Check sheet for the modelled part. Datum: model origin and axes. Units: mm. A direction names the side the tool comes from. Give positions to 0.01 mm unless a question says otherwise; leave off trailing zeros. Loops run counter-clockwise (first coordinate to the right, second up) from the corner with the lowest first, then second, coordinate; pieces in that order, holes last. Notation, with made-up numbers: M 24.5,29.25 L 56.5,29.25 A9 cw 56.5,38.25 Z; hole C -16,9.25 d5. An arc over 180 degrees is marked long. One line per question, with ' | ' between items. Start each with the question number.
from build123d import *

# Parameters (mm, degrees)
SKETCH1_W              = 127
SKETCH1_H              = 111.76
BASE_FLANGE1_DEPTH     = 1.5875
SKETCHED_START         = -63.5
SKETCHED_BEND1_DEPTH   = 127
SKETCHED_BEND1_2_DEPTH = 127
CUT_EXTRUDE2_START     = -2.3241
CUT_EXTRUDE2_OUTLINE_W = 17.78
CUT_EXTRUDE2_OUTLINE_H = 84
CUT_EXTRUDE2_DEPTH     = 2.3241
CUT_EXTRUDE1_REACH     = 106.317
SKETCH6_R              = 3.96875
CUT_EXTRUDE3_DEPTH     = 78.328235904
SKETCH34_W             = 31.75
SKETCH34_H             = 73.025
CUT_EXTRUDE5_DEPTH     = 2.54
CUT_EXTRUDE6_REACH     = 106.317
SKETCH49_W             = 17.78
SKETCH49_H             = 2.54


# Read off the part's stored shape, not the designer's step: Sketched Bend1, Cut-Extrude2
# Sheet-metal steps are written as plain solids
with BuildPart() as part:
    # Sketch1 → Base-Flange1 (new body)
    with BuildSketch(Plane.XY):
        Rectangle(SKETCH1_W, SKETCH1_H)
    extrude(amount=-BASE_FLANGE1_DEPTH)

    # Sketched Bend1 outline → Sketched Bend1 (cut)
    with BuildSketch(Plane.YZ.offset(SKETCHED_START)):
        with BuildLine():
            ThreePointArc((38.1, 0), (39.458217352, -0.438182071), (40.304282479, -1.5875))
            Line((40.304282479, -1.5875), (55.88, -1.5875))
            Line((55.88, -1.5875), (55.88, 0))
            Line((55.88, 0), (38.1, 0))
        make_face()
        with BuildLine():
            Line((-55.88, -1.5875), (-40.304282479, -1.5875))
            ThreePointArc((-40.304282479, -1.5875), (-39.458217352, -0.438182071), (-38.1, 0))
            Line((-38.1, 0), (-55.88, 0))
            Line((-55.88, 0), (-55.88, -1.5875))
        make_face()
    extrude(amount=SKETCHED_BEND1_DEPTH, mode=Mode.SUBTRACT)

    # Sketched Bend1 2 outline → Sketched Bend1 2 (add)
    with BuildSketch(Plane.YZ.offset(SKETCHED_START)):
        with BuildLine():
            ThreePointArc((38.1, -1.5875), (38.620854855, -1.803245145), (38.8366, -2.3241))
            Line((38.8366, -2.3241), (38.8366, -17.700231841))
            Line((38.8366, -17.700231841), (40.4241, -17.700231841))
            Line((40.4241, -17.700231841), (40.4241, -2.3241))
            ThreePointArc((40.4241, -2.3241), (40.393950056, -1.950959343), (40.304282479, -1.5875))
            Line((40.304282479, -1.5875), (38.1, -1.5875))
        make_face()
        with BuildLine():
            ThreePointArc((-38.8366, -2.3241), (-38.620854855, -1.803245145), (-38.1, -1.5875))
            Line((-38.1, -1.5875), (-40.304282479, -1.5875))
            ThreePointArc((-40.304282479, -1.5875), (-40.393950056, -1.950959343), (-40.4241, -2.3241))
            Line((-40.4241, -2.3241), (-40.4241, -17.700231841))
            Line((-40.4241, -17.700231841), (-38.8366, -17.700231841))
            Line((-38.8366, -17.700231841), (-38.8366, -2.3241))
        make_face()
    extrude(amount=SKETCHED_BEND1_2_DEPTH)

    # Cut-Extrude2 outline → Cut-Extrude2 (cut)
    with BuildSketch(Plane.XY.offset(CUT_EXTRUDE2_START)):
        with Locations((54.61, 0)):
            Rectangle(CUT_EXTRUDE2_OUTLINE_W, CUT_EXTRUDE2_OUTLINE_H)
    extrude(amount=CUT_EXTRUDE2_DEPTH, mode=Mode.SUBTRACT)

    # Cut-Extrude1: up to this face of the body (flat: up to its plane)
    cut_extrude1_end = Plane(part.part.faces().sort_by_distance((0, -40.4241, -10.012165921))[0])
    # Sketch6 → Cut-Extrude1 (cut, up to the picked face)
    with BuildSketch(Plane(origin=(0, 40.4241, 0), x_dir=(1, 0, 0), z_dir=(0, 1, 0)), mode=Mode.PRIVATE) as cut_extrude1_sk1:
        with Locations(Location((56.515, 10.4775, 0), (0, 0, 270))):
            Circle(SKETCH6_R)
    cut_extrude1_tool1 = split(extrude(cut_extrude1_sk1.sketch, amount=-CUT_EXTRUDE1_REACH, mode=Mode.PRIVATE), bisect_by=cut_extrude1_end, keep=Keep.BOTH, mode=Mode.PRIVATE)
    add(cut_extrude1_tool1.solids().sort_by(Axis((56.515, 40.4241, -10.4775), (0, -1, 0)))[0], mode=Mode.SUBTRACT)

    # Sketch13 → Cut-Extrude3 (cut, through all)
    with BuildSketch(Plane.XY):
        with BuildLine():
            ThreePointArc((45.72, 4.050728383), (44.765416013, 4.386244277), (43.76000011, 4.5))
            ThreePointArc((43.76000011, 4.5), (39.26000011, 0), (43.76000011, -4.5))
            ThreePointArc((43.76000011, -4.5), (44.765416013, -4.386244277), (45.72, -4.050728383))
            Line((45.72, -4.050728383), (45.72, 4.050728383))
        make_face()
        with BuildLine():
            ThreePointArc((48.26000011, 0), (47.572479586, 2.390606669), (45.72, 4.050728383))
            Line((45.72, 4.050728383), (45.72, -4.050728383))
            ThreePointArc((45.72, -4.050728383), (47.572479586, -2.390606669), (48.26000011, 0))
        make_face()
        with BuildLine():
            Line((45.72, 4.5), (43.76000011, 4.5))
            ThreePointArc((43.76000011, 4.5), (44.765416013, 4.386244277), (45.72, 4.050728383))
            Line((45.72, 4.050728383), (45.72, 4.5))
        make_face()
        with BuildLine():
            ThreePointArc((45.72, -4.050728383), (44.765416013, -4.386244277), (43.76000011, -4.5))
            Line((43.76000011, -4.5), (45.72, -4.5))
            Line((45.72, -4.5), (45.72, -4.050728383))
        make_face()
    extrude(amount=-CUT_EXTRUDE3_DEPTH, mode=Mode.SUBTRACT)

    # Sketch34 → Cut-Extrude5 (cut)
    with BuildSketch(Plane.XY):
        with Locations((-47.625, 0)):
            Rectangle(SKETCH34_W, SKETCH34_H)
    extrude(amount=-CUT_EXTRUDE5_DEPTH, mode=Mode.SUBTRACT)

    # Cut-Extrude6: up to this face of the body (flat: up to its plane)
    cut_extrude6_end = Plane(part.part.faces().sort_by_distance((-1.469322503, 40.4241, -10.00006779))[0])
    # Sketch49 → Cut-Extrude6 (cut, up to the picked face)
    with BuildSketch(Plane.XZ.offset(40.4241), mode=Mode.PRIVATE) as cut_extrude6_sk1:
        with Locations((54.61, -3.5941)):
            Rectangle(SKETCH49_W, SKETCH49_H)
    cut_extrude6_tool1 = split(extrude(cut_extrude6_sk1.sketch, amount=-CUT_EXTRUDE6_REACH, mode=Mode.PRIVATE), bisect_by=cut_extrude6_end, keep=Keep.BOTH, mode=Mode.PRIVATE)
    add(cut_extrude6_tool1.solids().sort_by(Axis((54.61, -40.4241, -3.5941), (0, 1, 0)))[0], mode=Mode.SUBTRACT)


solid = part.part
Q1. Cross-section at A-A (x = -44). Record the cut outline in (y, z).
Q2. Depth check by flat-ended pin: P1, Ø1.3, axis at x = -47, z = -1, coming from the -Y side; P2, Ø0.8, axis at x = -48, z = -1, coming from the +Y side; P3, Ø0.5, axis at x = 55, y = 39.5, coming from the +Z side; P4, Ø10, axis at x = 28, y = 4, coming from the +Z side. Enter the tip coordinate at first touch or a pass-through.
Q3. Access from +Z, -Z, +X, -X, +Y, -Y to the whole of each face (thin tool, end or side, straight path). Record for faces 1 (the flat face through (-63.5, -39, -9)), 2 (the flat face through (-1, 38.837, -10)).
Q4. Draft check along Y on faces 3 (the flat face through (-1, -38.837, -10)), 4 (the flat face through (-1, 40.424, -10)), 5 (the flat face through (45.72, -24, -1)), 6 (the flat face through (-1, -40.424, -10)). Enter one of: released by +Y, released by -Y, zero draft, split by the parting line, or undercut.
Q5. Cross-section at C-C (y = -9). Record the cut outline in (x, z).
Q6. Material ranges on probe 1 along Y at (x, z) = (-38.5, -12.25); probe 2 along Z at (x, y) = (-26, 3); probe 3 along X at (y, z) = (21.5, -1), recorded low to high. Write a range as from..to.
Q7. Cross-section at D-D (x = 37). Record the cut outline in (y, z).
Q8. Cross-section at B-B (x = 55). Record the cut outline in (y, z).
Solved:
1) outline: M -40.42,-17.7 L -38.84,-17.7 L -38.84,-2.32 A0.74 cw -38.1,-1.59 L -36.51,-1.59 L -36.51,0 L -38.1,0 A2.32 ccw -40.42,-2.32 Z; M 36.51,-1.59 L 38.1,-1.59 A0.74 cw 38.84,-2.32 L 38.84,-17.7 L 40.42,-17.7 L 40.42,-2.32 A2.32 ccw 38.1,0 L 36.51,0 Z
2) P1: stops at y = -40.32 | P2: stops at y = 40.23 | P3: stops at z = -4.86 | P4: stops at z = 0
3) face 1: +Z, -Z, -X, +Y, -Y | face 2: -Z, +X, -X
4) face 3: undercut | face 4: released by +Y | face 5: zero draft | face 6: released by -Y
5) outline: M -31.75,-1.59 L 45.72,-1.59 L 45.72,0 L -31.75,0 Z
6) probe 1: y = -40.42..-38.84, 38.84..40.42 | probe 2: z = -1.59..0 | probe 3: x = -31.75..45.72
7) outline: M -40.42,-17.7 L -38.84,-17.7 L -38.84,-2.32 A0.74 cw -38.1,-1.59 L 38.1,-1.59 A0.74 cw 38.84,-2.32 L 38.84,-17.7 L 40.42,-17.7 L 40.42,-2.32 A2.32 ccw 38.1,0 L -38.1,0 A2.32 ccw -40.42,-2.32 Z
8) outline: M -40.42,-17.7 L -38.84,-17.7 L -38.84,-14.15 L -40.42,-14.15 Z; M -40.42,-6.81 L -38.84,-6.81 L -38.84,-4.86 L -40.42,-4.86 Z; M 38.84,-17.7 L 40.42,-17.7 L 40.42,-14.15 L 38.84,-14.15 Z; M 38.84,-6.81 L 40.42,-6.81 L 40.42,-4.86 L 38.84,-4.86 Z
